Autodesk Inventor part; units mm, degrees
ref_plane "YZ Plane" through (0, 0, 0) normal (1, 0, 0) x (0, 1, 0)
ref_plane "XZ Plane" through (0, 0, 0) normal (0, 1, 0) x (-1, 0, 0)
ref_plane "XY Plane" through (0, 0, 0) normal (0, 0, 1) x (1, 0, 0)
sketch "Náčrt1" plane through (0, 0, 0) normal (0, 1, 0) x (-1, 0, 0)
  line L0 (0, 0) -> (177.8, 0)
  line L1 (177.8, 0) -> (177.8, 50.8)
  line L2 (177.8, 50.8) -> (0, 50.8)
  line L3 (0, 50.8) -> (0, 0)
  dimension "d0" = 50.8
  dimension "d1" = 177.8
extrude "Vysunutí1" add sketch "Náčrt1" along normal blind 2.54
sketch "Náčrt3" plane through (0, 0, 0) normal (0, -1, 0) x (1, 0, 0)
  line L0 (0, 0) -> (-177.8, 0)
  line L1 (-177.8, 50.8) -> (0, 50.8)
  line L2 (-177.8, 50.8) -> (-175.26, 50.8)
  line L3 (-175.26, 50.8) -> (-175.26, 2.54)
  line L4 (-175.26, 2.54) -> (-2.54, 2.54)
  line L5 (-2.54, 2.54) -> (-2.54, 50.8)
  line L6 (-2.54, 50.8) -> (0, 50.8)
  line L7 (0, 50.8) -> (0, 0)
  line L8 (0, 0) -> (-177.8, 0)
  line L9 (-177.8, 0) -> (-177.8, 50.8)
  line L10 (0, 0) -> (-177.8, 0)
  line L11 (-177.8, 50.8) -> (-175.26, 50.8)
  dimension "d23" = 2.54
  dimension "d24" = 2.54
  dimension "d25" = 2.54
extrude "Vysunutí2" add sketch "Náčrt3" along normal blind 6.35 contours L0 L9 L1 L3 L4 L5 L7
sketch "Náčrt4" plane through (0, -6.35, 0) normal (0, -1, 0) x (1, 0, 0)
  line L0 (0, 50.8) -> (-2.54, 50.8)
  line L1 (-2.54, 50.8) -> (-1.27, 50.8)
  line L2 (-1.27, 1.27) -> (-176.53, 1.27)
  line L3 (-176.53, 1.27) -> (-176.53, 50.8)
  line L4 (-176.53, 50.8) -> (-175.26, 50.8)
  line L5 (-175.26, 50.8) -> (-175.26, 2.54)
  line L6 (-175.26, 2.54) -> (-2.54, 2.54)
  line L7 (-2.54, 2.54) -> (-2.54, 50.8)
  line L8 (-1.27, 1.27) -> (-1.27, 50.8)
  line L9 (-177.8, 0) -> (0, 0)
  line L10 (-177.8, 50.8) -> (-177.8, 0)
  dimension "d26" = 1.27
  dimension "d27" = 1.27
extrude "Vysunutí3" add sketch "Náčrt4" along normal blind 1.27
sketch "Náčrt5" plane through (0, 0, 0) normal (0, -1, 0) x (1, 0, 0)
  line L0 (-2.54, 2.54) -> (-2.54, 50.8)
  line L1 (-175.26, 50.8) -> (-2.54, 50.8)
  line L2 (-175.26, 50.8) -> (-175.26, 2.54)
  line L3 (-175.26, 41.275) -> (-2.54, 41.275)
  line L4 (-2.54, 41.275) -> (-2.54, 39.37)
  line L5 (-2.54, 39.37) -> (-175.26, 39.37)
  line L6 (-175.26, 39.37) -> (-175.26, 41.275)
  line L7 (-175.26, 2.54) -> (-175.26, 50.8)
  line L8 (-175.26, 37.465) -> (-2.54, 37.465)
  line L9 (-2.54, 37.465) -> (-2.54, 35.56)
  line L10 (-2.54, 35.56) -> (-175.26, 35.56)
  line L11 (-175.26, 35.56) -> (-175.26, 37.465)
  line L12 (-175.26, 28.575) -> (-2.54, 28.575)
  line L13 (-2.54, 28.575) -> (-2.54, 26.67)
  line L14 (-2.54, 26.67) -> (-175.26, 26.67)
  line L15 (-175.26, 26.67) -> (-175.26, 28.575)
  line L16 (-175.26, 24.765) -> (-2.54, 24.765)
  line L17 (-2.54, 24.765) -> (-2.54, 22.86)
  line L18 (-2.54, 22.86) -> (-175.26, 22.86)
  line L19 (-175.26, 22.86) -> (-175.26, 24.765)
  line L20 (-175.26, 15.875) -> (-2.54, 15.875)
  line L21 (-2.54, 15.875) -> (-2.54, 13.97)
  line L22 (-2.54, 13.97) -> (-175.26, 13.97)
  line L23 (-175.26, 13.97) -> (-175.26, 15.875)
  line L24 (-175.26, 12.065) -> (-2.54, 12.065)
  line L25 (-2.54, 12.065) -> (-2.54, 10.16)
  line L26 (-2.54, 10.16) -> (-175.26, 10.16)
  line L27 (-175.26, 10.16) -> (-175.26, 12.065)
  point P0 (0, 0)
  dimension "d8" = 1.905
  dimension "d10" = 1.905
  dimension "d11" = 1.905
  dimension "d12" = 1.905
  dimension "d13" = 1.905
  dimension "d14" = 1.905
  dimension "d15" = 1.905
  dimension "d16" = 1.905
  dimension "d17" = 1.905
  dimension "d18" = 11.43
  dimension "d19" = 10.795
  dimension "d20" = 10.795
extrude "Vysunutí4" add sketch "Náčrt5" along normal blind 1.905 contours L26 L2 L24 L0 | L22 L2 L20 L0 | L18 L2 L16 L0 | L14 L2 L12 L0 | L10 L2 L8 L0 | L5 L2 L3 L0
sketch "Náčrt6" plane through (0, -1.905, 0) normal (0, -1, 0) x (1, 0, 0)
  line L0 (-2.54, 41.275) -> (-175.26, 41.275)
  line L1 (-175.26, 39.37) -> (-173.3599, 39.37)
  line L2 (-173.3599, 39.37) -> (-173.3599, 41.275)
  line L3 (-173.3599, 41.275) -> (-175.26, 41.275)
  line L4 (-175.26, 41.275) -> (-175.26, 39.37)
  line L5 (-2.54, 39.37) -> (-4.4571, 39.37)
  line L6 (-4.4571, 39.37) -> (-4.4571, 41.275)
  line L7 (-4.4571, 41.275) -> (-2.54, 41.275)
  line L8 (-2.54, 41.275) -> (-2.54, 39.37)
  point P0 (0, 0)
extrude "Vysunutí5" add sketch "Náčrt6" along normal up to surface (5.715 mm away)
sketch "Náčrt7" plane through (0, -1.905, 0) normal (0, -1, 0) x (1, 0, 0)
  line L0 (-175.26, 35.56) -> (-175.26, 37.465)
  line L1 (-175.26, 35.56) -> (-2.54, 35.56)
  line L2 (-2.54, 37.465) -> (-175.26, 37.465)
  line L3 (-175.26, 37.465) -> (-173.3424, 37.465)
  line L4 (-173.3424, 37.465) -> (-173.3424, 35.56)
  line L5 (-173.3424, 35.56) -> (-175.26, 35.56)
  line L6 (-175.26, 35.56) -> (-175.26, 37.465)
  line L7 (-2.54, 35.56) -> (-4.4396, 35.56)
  line L8 (-4.4396, 35.56) -> (-4.4396, 37.465)
  line L9 (-4.4396, 37.465) -> (-2.54, 37.465)
  line L10 (-2.54, 37.465) -> (-2.54, 35.56)
  point P0 (0, 0)
extrude "Vysunutí6" add sketch "Náčrt7" along normal up to surface (5.715 mm away) contours L0 L2 L4 L1 | L8 L2 L10 L1
sketch "Náčrt10" plane through (0, -1.905, 0) normal (0, -1, 0) x (1, 0, 0)
  line L0 (-2.54, 13.97) -> (-175.26, 13.97)
  line L1 (-175.26, 15.875) -> (-173.3527, 15.875)
  line L2 (-173.3527, 15.875) -> (-173.3527, 13.97)
  line L3 (-173.3527, 13.97) -> (-175.26, 13.97)
  line L4 (-175.26, 13.97) -> (-175.26, 15.875)
  line L5 (-2.54, 15.875) -> (-4.4457, 15.875)
  line L6 (-4.4457, 15.875) -> (-4.4457, 13.97)
  line L7 (-4.4457, 13.97) -> (-2.54, 13.97)
  line L8 (-2.54, 13.97) -> (-2.54, 15.875)
  point P0 (0, 0)
extrude "Vysunutí9" add sketch "Náčrt10" along normal up to surface (5.715 mm away)
sketch "Náčrt11" plane through (0, -1.905, 0) normal (0, -1, 0) x (1, 0, 0)
  line L0 (-175.26, 10.16) -> (-2.54, 10.16)
  line L1 (-175.26, 12.065) -> (-173.3599, 12.065)
  line L2 (-173.3599, 12.065) -> (-173.3599, 10.16)
  line L3 (-173.3599, 10.16) -> (-175.26, 10.16)
  line L4 (-175.26, 10.16) -> (-175.26, 12.065)
  line L5 (-2.54, 12.065) -> (-4.4431, 12.065)
  line L6 (-4.4431, 12.065) -> (-4.4431, 10.16)
  line L7 (-4.4431, 10.16) -> (-2.54, 10.16)
  line L8 (-2.54, 10.16) -> (-2.54, 12.065)
  point P0 (0, 0)
extrude "Vysunutí10" add sketch "Náčrt11" along normal up to surface (5.715 mm away)
sketch "Náčrt12" plane through (0, 0, 0) normal (0, -1, 0) x (1, 0, 0)
  line L0 (-2.54, 35.56) -> (-175.26, 35.56)
  line L1 (-175.26, 35.56) -> (-175.26, 28.575)
  ellipse E0 centre (-127, 32.0675) end of major axis (-116.84, 32.0675) minor radius 3.175
  line L2 (-175.26, 50.8) -> (-2.54, 50.8)
  ellipse E1 centre (-50.8, 32.0675) end of major axis (-40.64, 32.0675) minor radius 3.175
  point P0 (0, 0)
  dimension "d42" = 10.16
  dimension "d43" = 3.175
  dimension "d45" = 10.16
  dimension "d46" = 3.175
  dimension "d40" = 48.26
  dimension "d41" = 18.7325
  dimension "d44" = 76.2
  dimension "d47" = 0
extrude "Vysunutí11" add sketch "Náčrt12" along normal up to surface (7.62 mm away)
sketch "Náčrt13" plane through (-127, -7.62, 32.0675) normal (0, -1, 0) x (1, 0, 0)
  ellipse E0 centre (0, 0) end of major axis (-10.16, 0) minor radius 3.175
  circle A0 centre (0, 0) radius 0.9525
  point P0 (127, -32.0675)
  dimension "d50" = 1.905
extrude "Vysunutí12" cut sketch "Náčrt13" against normal through all contours A0
sketch "Náčrt14" plane through (-50.8, -7.62, 32.0675) normal (0, -1, 0) x (1, 0, 0)
  ellipse E0 centre (0, 0) end of major axis (-10.16, 0) minor radius 3.175
  circle A0 centre (0, 0) radius 0.9525
  point P0 (50.8, -32.0675)
  dimension "d53" = 1.905
extrude "Vysunutí13" cut sketch "Náčrt14" against normal through all contours A0
sketch "Náčrt15" plane through (0, 2.54, 0) normal (0, 1, 0) x (1, 0, 0)
  circle A0 centre (-50.8, -32.0675) radius 0.9525
  circle A1 centre (-127, -32.0675) radius 0.9525
  circle A2 centre (-127, -32.0675) radius 2.667
  circle A3 centre (-50.8, -32.0675) radius 2.667
  dimension "d56" = 5.334
  dimension "d57" = 5.334
extrude "Vysunutí14" cut sketch "Náčrt15" against normal blind 2.54
sketch "Náčrt16" plane through (0, -7.62, 0) normal (0, -1, 0) x (1, 0, 0)
  line L0 (-2.54, 2.54) -> (-175.26, 2.54)
  line L1 (-175.26, 2.54) -> (-175.26, 10.16)
  line L2 (-176.53, 1.27) -> (-1.27, 1.27)
  line L3 (-170.18, 2.54) -> (-149.86, 2.54)
  line L4 (-149.86, 2.54) -> (-149.86, 1.27)
  line L5 (-149.86, 1.27) -> (-170.18, 1.27)
  line L6 (-170.18, 1.27) -> (-170.18, 2.54)
  point P0 (0, 0)
  dimension "d60" = 20.32
  dimension "d61" = 25.4
extrude "Vysunutí15" cut sketch "Náčrt16" against normal up to surface (1.27 mm away)
properties part number "NavCom_Box_Upper_Part"
Build history of the part. All positions in model axes, mm. A direction names the side the tool comes from. Round coordinates to 2 decimals unless told otherwise and drop trailing zeros. Write each loop counter-clockwise with the first axis right and the second up, starting at its lowest first coordinate (ties: lowest second). Pieces come first, ordered by that corner, then holes. Notation, with made-up numbers: M 87,25.25 L 130,25.25 A24 ccw 130,48.25 Z; hole C -34.75,84 d4. An arc over 180 degrees is marked long. Answer as a JSON object with one key per item and string values. Group by question number.
(1) Flat gauge pin, fed straight in: pin 1 (2 mm diameter, centred on x = -108, z = 11, fed in from -Y) (3 decimals). Where does the tip first touch, or does it go through?
(2) Mould opens along Z. For faces 1 (the flat face through (-89, -6.35, 1)), 2 (the flat face through (-88, -1, 41.275)), 3 (the flat face through (-88, -2, 0)), 4 (the cylindrical face through (-52.916, 1.288, 33.69)) say: pulls with the +Z half, pulls with the -Z half, needs draft (parallel to the pull), parting line crosses it, or undercut.
(3) Which spindle directions (+Z, -Z, +X, -X, +Y, -Y) get a long thin tool onto all of the face, cutting with end or side? Do faces 5 (the cylindrical face through (-124.536, 1.288, 33.089)), 6 (the flat face through (-177.8, -2, 25)), 7 (the flat face through (-88, 0, 46)), 8 (the flat face through (-2.54, -4, 26)). Say none if no direction does.
(4) Drill centre lines: L1, parallel to Z at x = -50.8, y = -2 (1 decimal); L2, parallel to X at y = -3, z = 9; L3, parallel to Y at x = -37.5, z = 39.5 (3 decimals). Where is each one in solid material? Low to high.
(5) Cut at A-A (z = 19.5). Give the cut face in (x, y), and give its area (3 significant figures).
Responses:
{
 "1": {"pin 1": "stops at y = -1.905"},
 "2": {"face 1": "needs draft", "face 2": "pulls with the +Z half", "face 3": "pulls with the -Z half", "face 4": "undercut"},
 "3": {"face 5": "+Y", "face 6": "+Z, -Z, -X, +Y, -Y", "face 7": "+Z, -Y", "face 8": "-Y"},
 "4": {"L1": "z = 0 to 2.5, 28.9 to 31.1, 33 to 35.2", "L2": "x = -177.8 to -175.26, -2.54 to 0", "L3": "y = -1.905 to 2.54"},
 "5": {"outline": "M -177.8,-6.35 L -176.53,-6.35 L -176.53,-7.62 L -175.26,-7.62 L -175.26,0 L -2.54,0 L -2.54,-7.62 L -1.27,-7.62 L -1.27,-6.35 L 0,-6.35 L 0,2.54 L -177.8,2.54 Z", "area": "487 mm2"}
}
